from build123d import *

# Parameters (mm, degrees)
SKETCH1_W           = 54
SKETCH1_H           = 50
BOSS_EXTRUDE1_DEPTH = 2.5
SKETCH2_W           = 2.5
SKETCH2_H           = 50
BOSS_EXTRUDE2_DEPTH = 51
SKETCH3_R           = 11.25
CUT_EXTRUDE1_DEPTH  = 51
SKETCH4_W           = 35
SKETCH4_H           = 5
CUT_EXTRUDE2_DEPTH  = 51


with BuildPart() as part:
    # Sketch1 → Boss-Extrude1 (new body)
    with BuildSketch(Plane.XY):
        Rectangle(SKETCH1_W, SKETCH1_H)
    extrude(amount=BOSS_EXTRUDE1_DEPTH)

    # Sketch2 → Boss-Extrude2 (add)
    with BuildSketch(Plane.XY):
        with Locations((25.75, 0)):
            Rectangle(SKETCH2_W, SKETCH2_H)
    extrude(amount=BOSS_EXTRUDE2_DEPTH)

    # Sketch3 → Cut-Extrude1 (cut)
    with BuildSketch(Plane(origin=(0, 0, 0), x_dir=(0, 0, -1), z_dir=(1, 0, 0))):
        with Locations(Location((-30.25, 0, 0), (0, 0, 180))):
            Circle(SKETCH3_R)
    extrude(amount=CUT_EXTRUDE1_DEPTH, mode=Mode.SUBTRACT)

    # Sketch4 → Cut-Extrude2 (cut)
    with BuildSketch(Plane.XY):
        with Locations((-0.5, 15)):
            Rectangle(SKETCH4_W, SKETCH4_H)
        with Locations((-0.5, -15)):
            Rectangle(SKETCH4_W, SKETCH4_H)
    extrude(amount=CUT_EXTRUDE2_DEPTH, mode=Mode.SUBTRACT)


solid = part.part
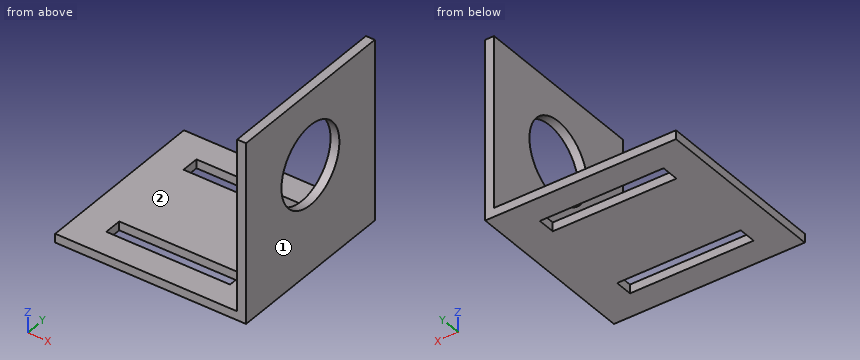
Source: CAD feature listing. Evaluate the final solid. Frame: model axes, mm. Face numbers are marked on the shaded views. A direction names the side the tool comes from. Round coordinates to 2 decimals unless told otherwise and drop trailing zeros. Loops run counter-clockwise (first coordinate to the right, second up) from the corner with the lowest first, then second, coordinate; pieces in that order, holes last. Notation, with made-up numbers: (-22.75, 17.25) -> (-6.75, 17.25) arc R15 ccw to (-6.75, 32.25) -> close; hole circle Ø2 at (64.5, -35.75). An arc over 180 degrees is marked (long way). Answer as a JSON object with one key per item and string values. Group by question number.
Q1. Contact query for flat-ended pins moving along their axis: P1, Ø24, axis at y = -5, z = 19, coming from the -X side; P2, Ø15, axis at x = 9.5, y = -5.5, coming from the +Z side; P3, Ø20, axis at y = 0, z = 30.25, coming from the -X side. Output: stop coordinate, or through.
Q2. Ray query, line 1 (Y direction, x = 25.7, z = 30.25); line 2 (X direction, y = -2, z = 17); line 3 (Z direction, x = 8.5, y = 9). Return the intervals inside material, ascending. Write a range as from..to.
Q3. Section query B-B (z = 30.25). Output: boundary loops of the cut face in (x, y), plus the area to 4 significant figures.
Q4. Access query for the marked faces 1 and 2. Directions: +Z, -Z, +X, -X, +Y, -Y. A direction counts if a zero-diameter tool reaches every point of the face in a straight line with its end or side. Return the directions, or none.
Q5. Section query C-C (x = 10.5). Output: boundary loops of the cut face in (y, z).
Q6. Section query D-D (y = 0). Output: boundary loops of the cut face in (x, z).
Q7. Section query A-A (y = -16). Output: boundary loops of the cut face in (x, z), plus the area to 3 significant figures.
Completed:
{
 "1": {"P1": "x = 24.5", "P2": "z = 2.5", "P3": "through"},
 "2": {"line 1": "-25..-11.25, 11.25..25", "line 2": "24.5..27", "line 3": "0..2.5"},
 "3": {"outline": "(24.5, -25) -> (27, -25) -> (27, -11.25) -> (24.5, -11.25) -> close; (24.5, 11.25) -> (27, 11.25) -> (27, 25) -> (24.5, 25) -> close", "area": "68.75 mm²"},
 "4": {"face 1": "+Z, -Z, +X, +Y, -Y", "face 2": "+Z, -X, +Y, -Y"},
 "5": {"outline": "(-25, 0) -> (-17.5, 0) -> (-17.5, 2.5) -> (-25, 2.5) -> close; (-12.5, 0) -> (12.5, 0) -> (12.5, 2.5) -> (-12.5, 2.5) -> close; (17.5, 0) -> (25, 0) -> (25, 2.5) -> (17.5, 2.5) -> close"},
 "6": {"outline": "(-27, 0) -> (27, 0) -> (27, 19) -> (24.5, 19) -> (24.5, 2.5) -> (-27, 2.5) -> close; (24.5, 41.5) -> (27, 41.5) -> (27, 51) -> (24.5, 51) -> close"},
 "7": {"outline": "(-27, 0) -> (-18, 0) -> (-18, 2.5) -> (-27, 2.5) -> close; (17, 0) -> (27, 0) -> (27, 51) -> (24.5, 51) -> (24.5, 2.5) -> (17, 2.5) -> close", "area": "169 mm²"}
}
